Geometry check sheet. Reference: the model listing, model coordinates, mm. Face numbers are marked on the shaded views. A direction names the side the tool comes from. Give positions to 0.01 mm unless a question says otherwise; leave off trailing zeros. Loops run counter-clockwise (first coordinate to the right, second up) from the corner with the lowest first, then second, coordinate; pieces in that order, holes last. Notation, with made-up numbers: (-7, 41) -> (48, 41) arc R23 cw to (48, 53) -> close; hole circle Ø5 at (27, 81.25). An arc over 180 degrees is marked (long way). One line per item, written item: value. Start each with the question number.
(1) Scan lines: line 1 along Z through (x, y) = (3.5, 7.5); line 2 along Z through (x, y) = (-7, -0.5); line 3 along Y through (x, z) = (4, 1). Record each from-to range of solid material in increasing order. Write a range as from..to.
(2) Tool access check on the marked faces 1 and 2. Record the directions out of +Z, -Z, +X, -X, +Y, -Y that give a thin tool (end or side, any length) a straight path to the whole face; none if there is none.
(3) Gauge pin test, flat ends, axial feed: pin 1 Ø2 at (y, z) = (6, 6) entering from -X; pin 2 Ø1 at (x, z) = (2.5, 7.5) entering from +Y; pin 3 Ø1.5 at (x, y) = (0.5, -8.5) entering from +Z. Record the tip position at first contact, or that the pin passes through.
(4) Sectioned sample at C-C, the plane z = 4.25. Record the cut outline in (x, y) (1 decimal).
(5) Sectioned sample at A-A, the plane y = 0. Record the cut outline in (x, z) (1 decimal).
(6) Sectioned sample at D-D, the plane z = 0.5. Record the cut outline in (x, y).
from build123d import *

# Parameters (mm, degrees)
CYLINDER_R     = 11.1125
CYLINDER_DEPTH = 3.96875
FILLET002_R    = 1.5875
FILLET003_R    = 1.5875
SKETCH001_R    = 7.9375
PAD001_DEPTH   = 1.5875
FILLET004_R    = 0.79375
SKETCH002_R    = 3.96875
PAD002_DEPTH   = 3.1
FILLET005_R    = 0.79375


with BuildPart() as part:
    # Cylinder → Cylinder (new body)
    with BuildSketch(Plane.XY):
        Circle(CYLINDER_R)
    extrude(amount=CYLINDER_DEPTH)

    # Fillet002
    fillet002_edges = [part.edges().sort_by_distance(p)[0] for p in [
        (-11.1125, 0, 3.96875),
    ]]
    fillet(fillet002_edges, radius=FILLET002_R)

    # Fillet003
    fillet003_edges = [part.edges().sort_by_distance(p)[0] for p in [
        (-11.1125, 0, 0),
    ]]
    fillet(fillet003_edges, radius=FILLET003_R)

    # Sketch001 → Pad001 (new body)
    with BuildSketch(Plane.XY.offset(3.96875)):
        Circle(SKETCH001_R)
    extrude(amount=PAD001_DEPTH)

    # Fillet004
    fillet004_edges = [part.edges().sort_by_distance(p)[0] for p in [
        (-7.9375, 0, 5.55625),
    ]]
    fillet(fillet004_edges, radius=FILLET004_R)

    # Sketch002 → Pad002 (new body)
    with BuildSketch(Plane.XY.offset(5.55625)):
        Circle(SKETCH002_R)
    extrude(amount=PAD002_DEPTH)

    # Fillet005
    fillet005_edges = [part.edges().sort_by_distance(p)[0] for p in [
        (-3.96875, 0, 8.65625),
    ]]
    fillet(fillet005_edges, radius=FILLET005_R)


solid = part.part
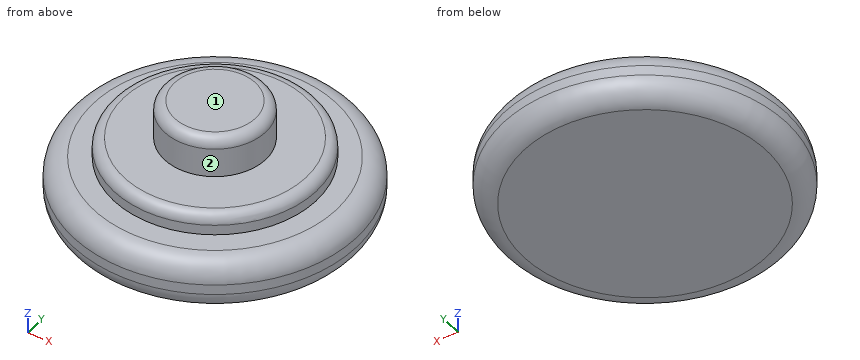
Calculated:
1. line 1: z = 0..3.97
1. line 2: z = 0..5.56
1. line 3: y = -10.25..10.25
2. face 1: +Z, +X, -X, +Y, -Y
2. face 2: +Z
3. pin 1: stops at x = -5.65
3. pin 2: stops at y = 3.43
3. pin 3: stops at z = 5.26
4. outline: circle Ø15.9 at (0, 0)
5. outline: (-11.1, 1.6) arc R1.6 ccw to (-9.5, 0) -> (9.5, 0) arc R1.6 ccw to (11.1, 1.6) -> (11.1, 2.4) arc R1.6 ccw to (9.5, 4) -> (7.9, 4) -> (7.9, 4.8) arc R0.8 ccw to (7.1, 5.6) -> (4, 5.6) -> (4, 7.9) arc R0.8 ccw to (3.2, 8.7) -> (-3.2, 8.7) arc R0.8 ccw to (-4, 7.9) -> (-4, 5.6) -> (-7.1, 5.6) arc R0.8 ccw to (-7.9, 4.8) -> (-7.9, 4) -> (-9.5, 4) arc R1.6 ccw to (-11.1, 2.4) -> close
6. outline: circle Ø21.36 at (0, 0)
